Autodesk Inventor part; units mm, degrees
ref_plane "YZ Plane" through (0, 0, 0) normal (1, 0, 0) x (0, 1, 0)
ref_plane "XZ Plane" through (0, 0, 0) normal (0, 1, 0) x (-1, 0, 0)
ref_plane "XY Plane" through (0, 0, 0) normal (0, 0, 1) x (1, 0, 0)
sketch "Sketch2" plane through (0, 0, 0) normal (0, 0, 1) x (1, 0, 0)
  line L0 (-20, -30) -> (20, -30)
  line L1 (20, -30) -> (20, 30)
  line L2 (20, 30) -> (-20, 30)
  line L3 (-20, 30) -> (-20, -30)
  line L4 (-20, -30) -> (20, 30) construction
  line L5 (20, -30) -> (-20, 30) construction
  line L6 (-10, 20) -> (10, 20) construction
  line L7 (10, 20) -> (10, 0) construction
  line L8 (10, 0) -> (10, -20) construction
  line L9 (10, -20) -> (-10, -20) construction
  line L10 (-10, -20) -> (-10, 0) construction
  line L11 (-10, 0) -> (10, 0) construction
  line L12 (-10, 20) -> (-10, 0) construction
  point P0 (0, 0)
  dimension "d0" = 40
  dimension "d1" = 60
  dimension "d2" = 20
  dimension "d3" = 20
extrude "Extrusion1" add sketch "Sketch2" along normal blind 5
hole "Hole1" at (-10, 20, 0) at (-10, 0, 0) at (-10, -20, 0) at (10, -20, 0) at (10, 0, 0) at (10, 20, 0) direction (0, 0, 1) diameter 5.5 end through all
fillet "Fillet1" radius 2 4 edges at (-20, 30, 2.5) (20, 30, 2.5) (-20, -30, 2.5) (20, -30, 2.5)
properties part number "4060Rect"
Part model, mm, in its own coordinate system. Round coordinates to 2 decimals unless told otherwise and drop trailing zeros. Write each loop counter-clockwise with the first axis right and the second up, starting at its lowest first coordinate (ties: lowest second). Pieces come first, ordered by that corner, then holes. Notation, with made-up numbers: M -34.75,36 L 8.25,36 A16 cw 8.25,40 Z; hole C 17.25,83.25 d4. An arc over 180 degrees is marked long. Answer as CSV lines item,"result". Start each with the question number.
1) Band-saw the part on D-D (x = 11). List the corners of the cut face in (y, z), then the cut area to 3 significant figures.
2) Drill centre lines: L1, parallel to Y at x = -10, z = 2.2; L2, parallel to X at y = 0, z = 1.7; L3, parallel to Y at x = 8, z = 1.2. Where is each one in solid material? Low to high.
3) Drop a flat-ended pin along its axis: pin 1 (5 mm diameter, centred on x = 10, y = -20, fed in from +Z). Give the stop position or say it passes through.
4) Mould opens along X. For faces 1 (the face through (-19.43, -29.4, 2.54)), 2 (the face through (0, -30, 2)), 3 (the face through (8.141, -2.027, 2.535)) say: +X half, -X half, draft (parallel to the pull), parting line (faces both ways), or undercut.
5) Band-saw the part on B-B (y = -20). List the corners of the cut face in (x, z).
6) Band-saw the part on C-C (z = 3.45). List the corners of the cut face in (x, y).
7) Band-saw the part on A-A (x = -10). List the corners of the cut face in (y, z).
Worked out:
1,outline,"M -30,0 L -22.56,0 L -22.56,5 L -30,5 Z; M -17.44,0 L -2.56,0 L -2.56,5 L -17.44,5 Z; M 2.56,0 L 17.44,0 L 17.44,5 L 2.56,5 Z; M 22.56,0 L 30,0 L 30,5 L 22.56,5 Z"
1,area,"223 mm²"
2,L1,"-30 to -22.75, -17.25 to -2.75, 2.75 to 17.25, 22.75 to 30"
2,L2,"-20 to -12.75, -7.25 to 7.25, 12.75 to 20"
2,L3,"-30 to -21.89, -18.11 to -1.89, 1.89 to 18.11, 21.89 to 30"
3,pin 1,"through"
4,face 1,"-X half"
4,face 2,"draft"
4,face 3,"undercut"
5,outline,"M -20,0 L -12.75,0 L -12.75,5 L -20,5 Z; M -7.25,0 L 7.25,0 L 7.25,5 L -7.25,5 Z; M 12.75,0 L 20,0 L 20,5 L 12.75,5 Z"
6,outline,"M -20,-28 A2 ccw -18,-30 L 18,-30 A2 ccw 20,-28 L 20,28 A2 ccw 18,30 L -18,30 A2 ccw -20,28 Z; hole C -10,-20 d5.5; hole C -10,0 d5.5; hole C -10,20 d5.5; hole C 10,-20 d5.5; hole C 10,0 d5.5; hole C 10,20 d5.5"
7,outline,"M -30,0 L -22.75,0 L -22.75,5 L -30,5 Z; M -17.25,0 L -2.75,0 L -2.75,5 L -17.25,5 Z; M 2.75,0 L 17.25,0 L 17.25,5 L 2.75,5 Z; M 22.75,0 L 30,0 L 30,5 L 22.75,5 Z"
